Can you work these out from the drawing? Everything is in mm from the part's minimum corner. Round coordinates to 2 decimals unless told otherwise and drop trailing zeros. Order: outer loops, then holes, each group sorted by start corner. A loop starts at its lowest first (then second) coordinate and runs counter-clockwise, first axis right, second up. Notation, with made-up numbers: (24.5, 83) -> (70.5, 83) arc R14 ccw to (70.5, 107) -> close; hole circle Ø7 at (13, 53). An arc over 180 degrees is marked (long way). One line per item, written item: value.
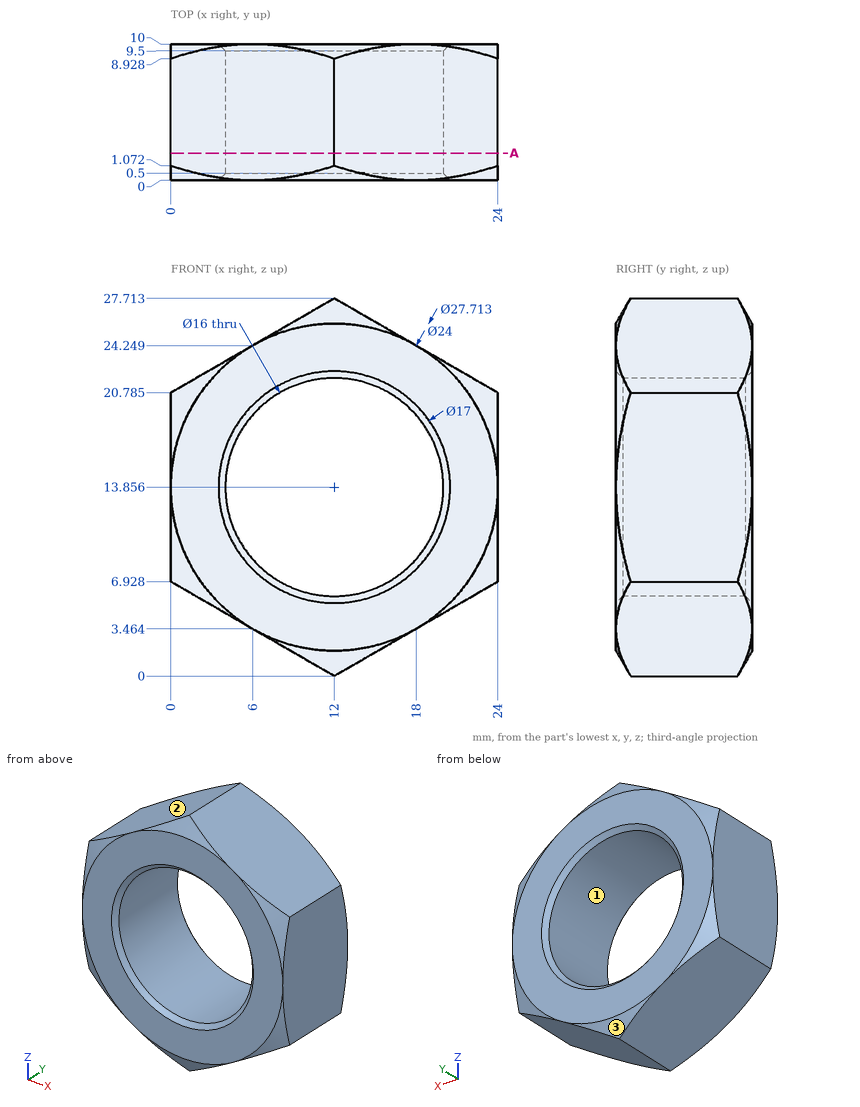
Q1. I want a section at A-A on y = 2. List the corners of the cut face in (x, z) for me (1 decimal).
Answers below:
outline: (0, 6.9) -> (12, 0) -> (24, 6.9) -> (24, 20.8) -> (12, 27.7) -> (0, 20.8) -> close; hole circle Ø16 at (12, 13.9)
Q2. Will these pins go through, and if not, where does the flat tip stop? pin 1 Ø6 at (x, y) = (5, 1) entering from -Z; pin 2 Ø2 at (x, y) = (5.5, 6) entering from -Z (1 decimal); pin 3 Ø3 at (x, z) = (10, 18) entering from +Y; pin 4 Ø6 at (x, y) = (17.5, 1.5) entering from +Z.
Answers below:
pin 1: z = 2.31
pin 2: z = 3.2
pin 3: through
pin 4: z = 26.27
Q3. We'd pull the mould along X, two halves only. Please class the marked faces 1, 2 and 3: released by +X, released by -X, zero draft, split by the parting line, or undercut.
Answers below:
face 1: undercut
face 2: released by -X
face 3: split by the parting line
Q4. Please list where these lines run through material, in increasing order: line 1 along Z through (x, y) = (13, 7.25) (1 decimal); line 2 along X through (y, z) = (6, 10.25); line 3 along Z through (x, y) = (4.75, 7.5) (1 decimal).
Answers below:
line 1: 0.6 to 5.9, 21.8 to 27.1
line 2: 0 to 4.86, 19.14 to 24
line 3: 4.2 to 10.5, 17.2 to 23.5
